```python
from build123d import *

# Parameters (mm, degrees)
SKETCH_W        = 120
SKETCH_H        = 80
PAD_DEPTH       = 80
SKETCH001_W     = 117
SKETCH001_H     = 77
POCKET_DEPTH    = 78.5
SKETCH002_W     = 32
SKETCH002_H     = 38
POCKET001_DEPTH = 2
SKETCH003_W     = 60
SKETCH003_H     = 10
POCKET002_DEPTH = 5
SKETCH004_W     = 60
SKETCH004_H     = 10
POCKET003_DEPTH = 5
POCKET004_DEPTH = 5
SKETCH006_W     = 4
SKETCH006_H     = 4
PAD001_DEPTH    = 1.5
SKETCH007_R     = 1.75
POCKET005_DEPTH = 1.5
SKETCH008_R     = 1.75
POCKET006_DEPTH = 1.5
SKETCH009_W     = 4
SKETCH009_H     = 4
PAD002_DEPTH    = 1.5
SKETCH010_R     = 1.75
POCKET007_DEPTH = 1.5
SKETCH011_R     = 1.75
POCKET008_DEPTH = 1.5
FILLET_R        = 1
FILLET001_R     = 1
FILLET002_R     = 1
FILLET003_R     = 1
SKETCH012_W     = 35
SKETCH012_H     = 1
PAD003_DEPTH    = 1
FILLET004_R     = 0.2
FILLET005_R     = 0.2
FILLET006_R     = 0.2
FILLET007_R     = 0.2
FILLET008_R     = 0.2
FILLET009_R     = 0.2
FILLET010_R     = 0.2
FILLET011_R     = 0.2
FILLET012_R     = 2
FILLET013_R     = 2
FILLET014_R     = 2
FILLET015_R     = 2
FILLET016_R     = 2
FILLET017_R     = 2
FILLET018_R     = 2
FILLET019_R     = 2
FILLET020_R     = 2
FILLET021_R     = 2
FILLET022_R     = 2
FILLET023_R     = 2
FILLET024_R     = 2
FILLET025_R     = 2
FILLET026_R     = 2
FILLET027_R     = 2


with BuildPart() as part:
    # Sketch → Pad (new body)
    with BuildSketch(Plane.XY):
        with Locations((3.133141, 0.368083)):
            Rectangle(SKETCH_W, SKETCH_H)
    extrude(amount=PAD_DEPTH)

    # Sketch001 (on Face6 of Pad) → Pocket (cut)
    with BuildSketch(Plane.XY.offset(80)):
        with Locations((3.133141, 0.368083)):
            Rectangle(SKETCH001_W, SKETCH001_H)
    extrude(amount=-POCKET_DEPTH, mode=Mode.SUBTRACT)

    # Sketch002 (on Face6 of Pocket) → Pocket001 (cut)
    with BuildSketch(Plane.XZ.offset(39.631917)):
        with Locations((3.133141, 40)):
            Rectangle(SKETCH002_W, SKETCH002_H)
    extrude(amount=-POCKET001_DEPTH, mode=Mode.SUBTRACT)

    # Sketch003 (on Face3 of Pocket001) → Pocket002 (cut)
    with BuildSketch(Plane.YZ.offset(63.133141)):
        with Locations((0.368083, 60)):
            Rectangle(SKETCH003_W, SKETCH003_H)
        with Locations((0.368083, 40)):
            Rectangle(SKETCH003_W, SKETCH003_H)
    extrude(amount=-POCKET002_DEPTH, mode=Mode.SUBTRACT)

    # Sketch004 (on Face2 of Pocket002) → Pocket003 (cut)
    with BuildSketch(Plane(origin=(-56.866859, 0, 0), x_dir=(0, -1, 0), z_dir=(-1, 0, 0))):
        with Locations((-0.368083, 60)):
            Rectangle(SKETCH004_W, SKETCH004_H)
        with Locations((-0.368083, 40)):
            Rectangle(SKETCH004_W, SKETCH004_H)
    extrude(amount=-POCKET003_DEPTH, mode=Mode.SUBTRACT)

    # Sketch005 (on Face3 of Pocket003) → Pocket004 (cut)
    with BuildSketch(Plane.YZ.offset(63.133141)):
        with BuildLine():
            Line((26.368083, 11), (26.368083, 5))
            Line((26.368083, 5), (35.368083, 5))
            Line((35.368083, 5), (35.368083, 11))
            ThreePointArc((35.368083, 11), (30.868083, 15.5), (26.368083, 11))
        make_face()
    extrude(amount=-POCKET004_DEPTH, mode=Mode.SUBTRACT)

    # Sketch006 (on Face27 of Pocket004) → Pad001 (join)
    with BuildSketch(Plane.XZ.offset(-38.868083)):
        with Locations((-33.366859, 78)):
            Rectangle(SKETCH006_W, SKETCH006_H)
        with Locations((39.633141, 78)):
            Rectangle(SKETCH006_W, SKETCH006_H)
    extrude(amount=PAD001_DEPTH)

    # Sketch007 (on Face44 of Pad001) → Pocket005 (cut)
    with BuildSketch(Plane.XZ.offset(-37.368083)):
        with Locations((-33.366859, 78)):
            Circle(SKETCH007_R)
    extrude(amount=-POCKET005_DEPTH, mode=Mode.SUBTRACT)

    # Sketch008 (on Face45 of Pocket005) → Pocket006 (cut)
    with BuildSketch(Plane.XZ.offset(-37.368083)):
        with Locations((39.633141, 78)):
            Circle(SKETCH008_R)
    extrude(amount=-POCKET006_DEPTH, mode=Mode.SUBTRACT)

    # Sketch009 (on Face31 of Pocket006) → Pad002 (join)
    with BuildSketch(Plane(origin=(0, -38.131917, 0), x_dir=(-1, 0, 0), z_dir=(0, 1, 0))):
        with Locations((-39.633141, 78)):
            Rectangle(SKETCH009_W, SKETCH009_H)
        with Locations((33.366859, 78)):
            Rectangle(SKETCH009_W, SKETCH009_H)
    extrude(amount=PAD002_DEPTH)

    # Sketch010 (on Face54 of Pad002) → Pocket007 (cut)
    with BuildSketch(Plane(origin=(0, -36.631917, 0), x_dir=(-1, 0, 0), z_dir=(0, 1, 0))):
        with Locations((-39.633141, 78)):
            Circle(SKETCH010_R)
    extrude(amount=-POCKET007_DEPTH, mode=Mode.SUBTRACT)

    # Sketch011 (on Face55 of Pocket007) → Pocket008 (cut)
    with BuildSketch(Plane(origin=(0, -36.631917, 0), x_dir=(-1, 0, 0), z_dir=(0, 1, 0))):
        with Locations((33.366859, 78)):
            Circle(SKETCH011_R)
    extrude(amount=-POCKET008_DEPTH, mode=Mode.SUBTRACT)

    # Fillet
    fillet_edges = [part.edges().sort_by_distance(p)[0] for p in [
        (-12.866859, -38.881917, 21),
    ]]
    fillet(fillet_edges, radius=FILLET_R)

    # Fillet001
    fillet001_edges = [part.edges().sort_by_distance(p)[0] for p in [
        (19.133141, -38.881917, 21),
    ]]
    fillet(fillet001_edges, radius=FILLET001_R)

    # Fillet002
    fillet002_edges = [part.edges().sort_by_distance(p)[0] for p in [
        (19.133141, -38.881917, 59),
    ]]
    fillet(fillet002_edges, radius=FILLET002_R)

    # Fillet003
    fillet003_edges = [part.edges().sort_by_distance(p)[0] for p in [
        (-12.866859, -38.881917, 59),
    ]]
    fillet(fillet003_edges, radius=FILLET003_R)

    # Sketch012 (on Face14 of Fillet003) → Pad003 (join)
    with BuildSketch(Plane(origin=(0, -38.131917, 0), x_dir=(-1, 0, 0), z_dir=(0, 1, 0))):
        with Locations((-3.133141, 19.5)):
            Rectangle(SKETCH012_W, SKETCH012_H)
    extrude(amount=PAD003_DEPTH)

    # Fillet004
    fillet004_edges = [part.edges().sort_by_distance(p)[0] for p in [
        (-35.366859, -36.631917, 78),
    ]]
    fillet(fillet004_edges, radius=FILLET004_R)

    # Fillet005
    fillet005_edges = [part.edges().sort_by_distance(p)[0] for p in [
        (-31.366859, -36.631917, 78),
    ]]
    fillet(fillet005_edges, radius=FILLET005_R)

    # Fillet006
    fillet006_edges = [part.edges().sort_by_distance(p)[0] for p in [
        (37.633141, -36.631917, 78),
    ]]
    fillet(fillet006_edges, radius=FILLET006_R)

    # Fillet007
    fillet007_edges = [part.edges().sort_by_distance(p)[0] for p in [
        (41.633141, -36.631917, 78),
    ]]
    fillet(fillet007_edges, radius=FILLET007_R)

    # Fillet008
    fillet008_edges = [part.edges().sort_by_distance(p)[0] for p in [
        (-35.366859, 37.368083, 78),
    ]]
    fillet(fillet008_edges, radius=FILLET008_R)

    # Fillet009
    fillet009_edges = [part.edges().sort_by_distance(p)[0] for p in [
        (-31.366859, 37.368083, 78),
    ]]
    fillet(fillet009_edges, radius=FILLET009_R)

    # Fillet010
    fillet010_edges = [part.edges().sort_by_distance(p)[0] for p in [
        (37.633141, 37.368083, 78),
    ]]
    fillet(fillet010_edges, radius=FILLET010_R)

    # Fillet011
    fillet011_edges = [part.edges().sort_by_distance(p)[0] for p in [
        (41.633141, 37.368083, 78),
    ]]
    fillet(fillet011_edges, radius=FILLET011_R)

    # Fillet012
    fillet012_edges = [part.edges().sort_by_distance(p)[0] for p in [
        (62.383141, 30.368083, 65),
    ]]
    fillet(fillet012_edges, radius=FILLET012_R)

    # Fillet013
    fillet013_edges = [part.edges().sort_by_distance(p)[0] for p in [
        (62.383141, 30.368083, 55),
    ]]
    fillet(fillet013_edges, radius=FILLET013_R)

    # Fillet014
    fillet014_edges = [part.edges().sort_by_distance(p)[0] for p in [
        (62.383141, 30.368083, 35),
    ]]
    fillet(fillet014_edges, radius=FILLET014_R)

    # Fillet015
    fillet015_edges = [part.edges().sort_by_distance(p)[0] for p in [
        (62.383141, 30.368083, 45),
    ]]
    fillet(fillet015_edges, radius=FILLET015_R)

    # Fillet016
    fillet016_edges = [part.edges().sort_by_distance(p)[0] for p in [
        (62.383141, -29.631917, 35),
    ]]
    fillet(fillet016_edges, radius=FILLET016_R)

    # Fillet017
    fillet017_edges = [part.edges().sort_by_distance(p)[0] for p in [
        (62.383141, -29.631917, 55),
    ]]
    fillet(fillet017_edges, radius=FILLET017_R)

    # Fillet018
    fillet018_edges = [part.edges().sort_by_distance(p)[0] for p in [
        (62.383141, -29.631917, 45),
    ]]
    fillet(fillet018_edges, radius=FILLET018_R)

    # Fillet019
    fillet019_edges = [part.edges().sort_by_distance(p)[0] for p in [
        (62.383141, -29.631917, 65),
    ]]
    fillet(fillet019_edges, radius=FILLET019_R)

    # Fillet020
    fillet020_edges = [part.edges().sort_by_distance(p)[0] for p in [
        (-56.116859, -29.631917, 55),
    ]]
    fillet(fillet020_edges, radius=FILLET020_R)

    # Fillet021
    fillet021_edges = [part.edges().sort_by_distance(p)[0] for p in [
        (-56.116859, -29.631917, 35),
    ]]
    fillet(fillet021_edges, radius=FILLET021_R)

    # Fillet022
    fillet022_edges = [part.edges().sort_by_distance(p)[0] for p in [
        (-56.116859, -29.631917, 45),
    ]]
    fillet(fillet022_edges, radius=FILLET022_R)

    # Fillet023
    fillet023_edges = [part.edges().sort_by_distance(p)[0] for p in [
        (-56.116859, -29.631917, 65),
    ]]
    fillet(fillet023_edges, radius=FILLET023_R)

    # Fillet024
    fillet024_edges = [part.edges().sort_by_distance(p)[0] for p in [
        (-56.116859, 30.368083, 55),
    ]]
    fillet(fillet024_edges, radius=FILLET024_R)

    # Fillet025
    fillet025_edges = [part.edges().sort_by_distance(p)[0] for p in [
        (-56.116859, 30.368083, 35),
    ]]
    fillet(fillet025_edges, radius=FILLET025_R)

    # Fillet026
    fillet026_edges = [part.edges().sort_by_distance(p)[0] for p in [
        (-56.116859, 30.368083, 65),
    ]]
    fillet(fillet026_edges, radius=FILLET026_R)

    # Fillet027
    fillet027_edges = [part.edges().sort_by_distance(p)[0] for p in [
        (-56.116859, 30.368083, 45),
    ]]
    fillet(fillet027_edges, radius=FILLET027_R)


solid = part.part
```
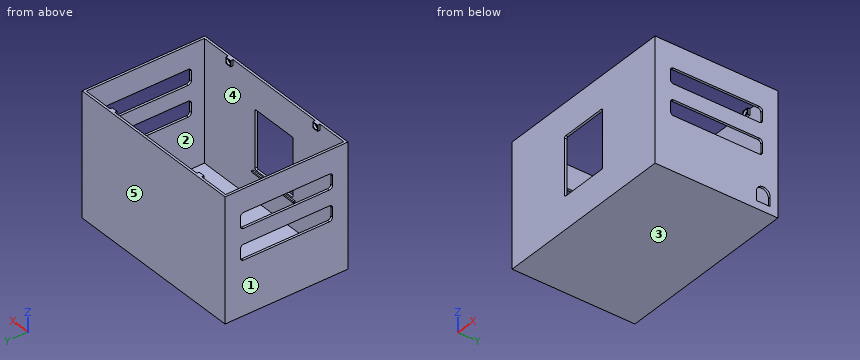
Input: part model. Units: mm. Frame: model coordinates. Face numbers are marked on the shaded views. A direction names the side the tool comes from. Coordinates: 2 decimals unless noted, no trailing zeros. Loops run counter-clockwise (first coordinate to the right, second up) from the corner with the lowest first, then second, coordinate; pieces in that order, holes last. Notation, with made-up numbers: M 29,22.25 L 44,22.25 A18 cw 44,28.25 Z; hole C -26,-35 d3. An arc over 180 degrees is marked long. One line per item, written item: value.
(1) Line query: line 1 along X through (y, z) = (-37, 78); line 2 along Y through (x, z) = (53.5, 9.5); line 3 along X through (y, z) = (16, 69). Output: solid intervals per line, ascending. Write a range as from..to.
Filled in:
line 1: -56.87..-55.37, -35.37..-35.12, -31.62..-31.37, 37.63..37.88, 41.38..41.63, 61.63..63.13
line 2: -39.63..-38.13, 38.87..40.37
line 3: -56.87..-55.37, 61.63..63.13
(2) Reachability of the marked faces 1 and 2 from +Z, -Z, +X, -X, +Y, -Y: full face, straight path, thin tool, end or side. Return the list, or none.
Filled in:
face 1: +Z, -Z, -X, +Y, -Y
face 2: +Z
(3) Pin query (flat end, axial travel): pin 1 (12 mm diameter, centred on x = -44.5, y = 17.5, fed in from +Z). Return the tip coordinate at first contact, or that it passes through.
Filled in:
pin 1: z = 1.5
(4) Section A-A (x = -0.5). Output: boundary loops of the cut face in (y, z).
Filled in:
outline: M -39.63,0 L 40.37,0 L 40.37,80 L 38.87,80 L 38.87,1.5 L -38.13,1.5 L -38.13,19 L -37.13,19 L -37.13,20 L -38.13,20 L -38.13,21 L -39.63,21 Z; M -39.63,59 L -38.13,59 L -38.13,80 L -39.63,80 Z
(5) Section B-B (z = 39). Output: boundary loops of the cut face in (x, y).
Filled in:
outline: M -56.87,-39.63 L -12.87,-39.63 L -12.87,-38.13 L -55.37,-38.13 L -55.37,-29.63 L -56.87,-29.63 Z; M -56.87,30.37 L -55.37,30.37 L -55.37,38.87 L 61.63,38.87 L 61.63,30.37 L 63.13,30.37 L 63.13,40.37 L -56.87,40.37 Z; M 19.13,-39.63 L 63.13,-39.63 L 63.13,-29.63 L 61.63,-29.63 L 61.63,-38.13 L 19.13,-38.13 Z
(6) Section D-D (z = 25.5). Output: boundary loops of the cut face in (x, y).
Filled in:
outline: M -56.87,-39.63 L -12.87,-39.63 L -12.87,-38.13 L -55.37,-38.13 L -55.37,38.87 L 61.63,38.87 L 61.63,-38.13 L 19.13,-38.13 L 19.13,-39.63 L 63.13,-39.63 L 63.13,40.37 L -56.87,40.37 Z
(7) Section C-C (y = -20). Output: boundary loops of the cut face in (x, z).
Filled in:
outline: M -56.87,0 L 63.13,0 L 63.13,35 L 61.63,35 L 61.63,1.5 L -55.37,1.5 L -55.37,35 L -56.87,35 Z; M -56.87,45 L -55.37,45 L -55.37,55 L -56.87,55 Z; M -56.87,65 L -55.37,65 L -55.37,80 L -56.87,80 Z; M 61.63,45 L 63.13,45 L 63.13,55 L 61.63,55 Z; M 61.63,65 L 63.13,65 L 63.13,80 L 61.63,80 Z
(8) Pull-direction query (Z, two-part tool) for the marked faces 3, 4 and 5; classes: +Z half, -Z half, draft (parallel to the pull), parting line (faces both ways), or undercut.
Filled in:
face 3: -Z half
face 4: undercut
face 5: draft
